The model under review builds one solid part; all positions refer to its coordinate system, in mm. A direction names the side the tool comes from. Coordinates: 2 decimals unless noted, no trailing zeros. Loops run counter-clockwise (first coordinate to the right, second up) from the corner with the lowest first, then second, coordinate; pieces in that order, holes last. Notation, with made-up numbers: (51.25, -37) - (77.25, -37) arc R23 cw to (77.25, -29) - close; hole circle Ø5 at (14, 79.25). An arc over 180 degrees is marked (long way). Answer in a Markdown table with one row per item. Add a question column.
(1) Mouldability with a two-part tool opening along Z and no side actions: class faces 4 (the cylindrical face through (-19.14, 3.45, -9.1)), 5 (the cylindrical face through (-16.597, 0.986, 0.158)), 6 (the cylindrical face through (16.434, 0.986, 1.081)), 7 (the cylindrical face through (-19.14, 3.45, 9.1)) as +Z half, -Z half, draft (parallel to the pull), parting line (faces both ways), or undercut.
(2) We need section D-D on x = 0. Write out the cut boundary in (y, z).
(3) We need section C-C on y = 5. Write out the cut boundary in (x, z), plus the area to 3 significant figures.
(4) We need section B-B on x = -13. Write out the cut boundary in (y, z).
(5) Machinability: for faces 1 (the flat face through (0, 4, 10)), 2 (the cylindrical face through (0, 2, -4)), 3 (the flat face through (-11, 2, -2)), which of the approach directions +Z, -Z, +X, -X, +Y, -Y give a long, thin tool a straight path to every point of the face, cutting with its end or side? Answer none if there is none.
(6) We need section A-A on z = 0. Write out the cut boundary in (x, y), plus the area to 3 significant figures.
(7) For line 1 along Z through (x, y) = (13, 4.1); line 2 along Z through (x, y) = (-13, 1.05); line 3 along X through (y, z) = (6.5, -0.75), list the stretches that pass through material, from the lowest coordinate up.
(8) For P1, Ø3.5, axis at x = -14, z = -0.5, coming from the -Y side; P2, Ø2.5, axis at x = -13, z = 0, coming from the -Y side; P3, Ø4, axis at x = 1, y = 4.5, coming from the -Z side; P4, Ø6.5, axis at x = 13, z = 0, coming from the +Y side, all flat-tipped, find the tip position at first contact; note any pin that passes through.
from build123d import *

# Parameters (mm, degrees)
PAD_DEPTH       = 10
SKETCH001_R     = 2.1
POCKET_DEPTH    = 10
FILLET_R        = 3
SKETCH002_R     = 3.6
POCKET001_DEPTH = 2
PAD001_DEPTH    = 8


with BuildPart() as part:
    # Sketch → Pad (new body, symmetric)
    with BuildSketch(Plane.XY):
        with BuildLine():
            Line((-20, 7), (-20, 0))
            Line((-20, 0), (20, 0))
            Line((20, 0), (20, 7))
            Line((20, 7), (5, 7))
            ThreePointArc((-5, 7), (0, 2), (5, 7))
            Line((-20, 7), (-5, 7))
        make_face()
    extrude(amount=PAD_DEPTH, both=True)

    # Sketch001 → Pocket (cut)
    with BuildSketch(Plane.XZ):
        with Locations((-13, 0)):
            Circle(SKETCH001_R)
        with Locations((13, 0)):
            Circle(SKETCH001_R)
    extrude(amount=-POCKET_DEPTH, mode=Mode.SUBTRACT)

    # Fillet
    fillet_edges = [part.edges().sort_by_distance(p)[0] for p in [
        (-20, 3.5, -10),
        (20, 3.5, -10),
        (-20, 3.5, 10),
        (20, 3.5, 10),
    ]]
    fillet(fillet_edges, radius=FILLET_R)

    # Sketch002 → Pocket001 (cut)
    with BuildSketch(Plane.XZ):
        with Locations((-13, 0)):
            Circle(SKETCH002_R)
        with Locations((13, 0)):
            Circle(SKETCH002_R)
    extrude(amount=-POCKET001_DEPTH, mode=Mode.SUBTRACT)

    # Sketch003 → Pad001 (new body)
    with BuildSketch(Plane.XY.offset(10)):
        with BuildLine():
            ThreePointArc((-5, 7), (0, 2), (5, 7))
            Line((-5, 7), (5, 7))
        make_face()
    extrude(amount=-PAD001_DEPTH)


solid = part.part
Outcome:
| question | item | result |
|---|---|---|
| 1 | face 4 | -Z half |
| 1 | face 5 | undercut |
| 1 | face 6 | undercut |
| 1 | face 7 | +Z half |
| 2 | outline | (0, -10) - (2, -10) - (2, 2) - (7, 2) - (7, 10) - (0, 10) - close |
| 3 | outline | (-20, -7) arc R3 ccw to (-17, -10) - (-4.58, -10) - (-4.58, 2) - (4.58, 2) - (4.58, -10) - (17, -10) arc R3 ccw to (20, -7) - (20, 7) arc R3 ccw to (17, 10) - (-17, 10) arc R3 ccw to (-20, 7) - close; hole circle Ø4.2 at (-13, 0); hole circle Ø4.2 at (13, 0) |
| 3 | area | 655 mm² |
| 4 | outline | (0, -10) - (7, -10) - (7, -2.1) - (2, -2.1) - (2, -3.6) - (0, -3.6) - close; (0, 3.6) - (2, 3.6) - (2, 2.1) - (7, 2.1) - (7, 10) - (0, 10) - close |
| 5 | face 1 | +Z, +X, -X, +Y, -Y |
| 5 | face 2 | -Z, +Y |
| 5 | face 3 | -Y |
| 6 | outline | (-20, 0) - (-16.6, 0) - (-16.6, 2) - (-15.1, 2) - (-15.1, 7) - (-20, 7) - close; (-10.9, 2) - (-9.4, 2) - (-9.4, 0) - (9.4, 0) - (9.4, 2) - (10.9, 2) - (10.9, 7) - (5, 7) arc R5 cw to (-5, 7) - (-10.9, 7) - close; (15.1, 2) - (16.6, 2) - (16.6, 0) - (20, 0) - (20, 7) - (15.1, 7) - close |
| 6 | area | 170 mm² |
| 7 | line 1 | -10 to -2.1, 2.1 to 10 |
| 7 | line 2 | -10 to -3.6, 3.6 to 10 |
| 7 | line 3 | -20 to -14.96, -11.04 to -4.97, 4.97 to 11.04, 14.96 to 20 |
| 8 | P1 | y = 2 |
| 8 | P2 | through |
| 8 | P3 | z = 2 |
| 8 | P4 | y = 7 |
